from build123d import *

# Parameters (mm, degrees)
CUT_EXTRUDE1_DEPTH       = 35
SKETCH3_R                = 6.25
CUT_EXTRUDE2_DEPTH       = 35
BOSS_EXTRUDE1_REACH      = 79.604
BOSS_EXTRUDE1_END_RADIUS = 23.432556387
SKETCH4_R                = 7.25
SKETCH4_R_2              = 6.25


with BuildPart() as part:
    # Sketch1 → Revolve1 (revolve)
    with BuildSketch(Plane.XY, mode=Mode.PRIVATE) as revolve1_sk:
        with BuildLine():
            Line((25.432556387, 0), (25.432556387, 41.5))
            Line((25.432556387, 41.5), (22.932556387, 41.5))
            Line((22.932556387, 41.5), (22.932556387, 44))
            Line((22.932556387, 44), (25.432556387, 44))
            Line((25.432556387, 44), (25.432556387, 47))
            Line((25.432556387, 47), (22.932556387, 47))
            Line((22.932556387, 47), (22.932556387, 49.5))
            Line((22.932556387, 49.5), (25.432556387, 49.5))
            Line((25.432556387, 49.5), (25.432556387, 54.5))
            ThreePointArc((25.432556387, 54.5), (13.510221664, 61.275659188), (0, 63.626304471))
            Line((0, 63.626304471), (0, 61.626304471))
            ThreePointArc((0, 61.626304471), (12.394048382, 59.548269405), (23.432556387, 53.541439456))
            Line((23.432556387, 53.541439456), (23.432556387, 51.5))
            Line((23.432556387, 51.5), (20.932556387, 51.5))
            Line((20.932556387, 51.5), (20.932556387, 45.5))
            Line((20.932556387, 45.5), (20.932556387, 39.5))
            Line((20.932556387, 39.5), (23.432556387, 39.5))
            Line((23.432556387, 39.5), (23.432556387, 0))
            Line((23.432556387, 0), (25.432556387, 0))
        make_face()
    revolve(revolve1_sk.sketch.rotate(Axis((0, 0, 0), (0, 1, 0)), 90), axis=Axis((0, 0, 0), (0, 1, 0)))

    # Sketch2 → Cut-Extrude1 (cut, symmetric)
    with BuildSketch(Plane(origin=(0, 0, 0), x_dir=(0, 0, -1), z_dir=(1, 0, 0))):
        with BuildLine():
            Line((-19, 0), (19, 0))
            ThreePointArc((19, 0), (0, 10), (-19, 0))
        make_face()
    extrude(amount=CUT_EXTRUDE1_DEPTH, both=True, mode=Mode.SUBTRACT)

    # Sketch3 → Cut-Extrude2 (cut, symmetric)
    with BuildSketch(Plane.XY):
        with Locations((0, 31.626304471)):
            Circle(SKETCH3_R)
    extrude(amount=CUT_EXTRUDE2_DEPTH, both=True, mode=Mode.SUBTRACT)

    # Boss-Extrude1: up to this cylinder (the profile starts inside it)
    boss_extrude1_end = Plane(origin=(0, 31.626304, 0), z_dir=(0, -1, 0)) * Cylinder(BOSS_EXTRUDE1_END_RADIUS, 207.073112775, mode=Mode.PRIVATE)
    # Sketch4 → Boss-Extrude1 (add, up to the surface)
    with BuildSketch(Plane.XY.offset(11), mode=Mode.PRIVATE) as boss_extrude1_sk1:
        with Locations(Location((0, 31.626304471, 0), (0, 0, 180))):
            Circle(SKETCH4_R)
        with Locations((0, 31.626304471)):
            Circle(SKETCH4_R_2, mode=Mode.SUBTRACT)
    boss_extrude1_tool1 = extrude(boss_extrude1_sk1.sketch, amount=BOSS_EXTRUDE1_REACH, mode=Mode.PRIVATE) & boss_extrude1_end
    boss_extrude1 = boss_extrude1_tool1.solids().sort_by_distance((7.044939, 31.626304, 11))[0]
    add(boss_extrude1)

    # Mirror1: Boss-Extrude1 across plane
    add(boss_extrude1.mirror(Plane.XY))


solid = part.part
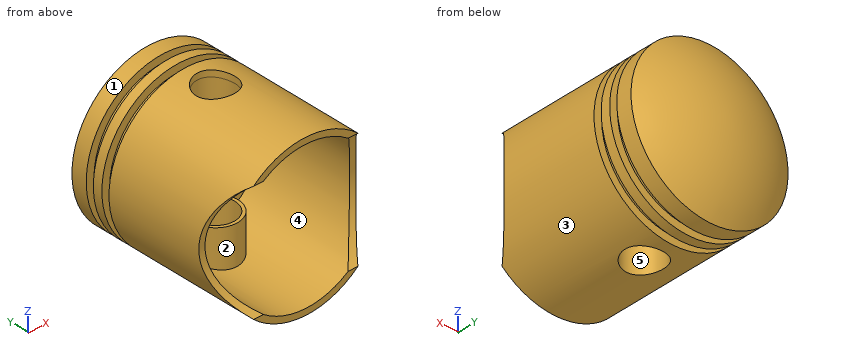
Part model, mm, in its own coordinate system. Face numbers are marked on the shaded views. A direction names the side the tool comes from. Coordinates: 2 decimals unless noted, no trailing zeros. Use a Markdown table: item, result. Add a question column.
Q1. Cut at A-A (z = 13.5). Give the number of separate pieces and of enclosed holes in the cut face, and give its area (3 significant figures).
Q2. Probe L1, parallel to X at y = 52.7, z = 0; L2, parallel to Y at x = 0, z = 24.2; L3, parallel to Y at x = 0, z = 24. List the from-to ranges inside material, lowest first.
Q3. Pin check, flat tips, straight feed: P1, Ø6, axis at x = -17, y = 10.5, coming from the +Z side; P2, Ø15.5, axis at x = 9, z = -3, coming from the -Y side; P3, Ø6, axis at x = -18.5, y = 24.5, coming from the -Z side; P4, Ø15.5, axis at x = 1, z = 1, coming from the +Y side. Stop position of each tip, or through.
Q4. Mould opens along Z. For the marked faces 3, 4 and 5 say: +Z half, -Z half, draft (parallel to the pull), parting line (faces both ways), or undercut.
Q5. Which spindle directions (+Z, -Z, +X, -X, +Y, -Y) get a long thin tool onto all of the face, cutting with end or side? Do the marked faces 1 and 2. Say none if no direction does.
Worked out:
| question | item | result |
|---|---|---|
| 1 | separate pieces | 2 |
| 1 | enclosed holes | 1 |
| 1 | area | 412 mm2 |
| 2 | L1 | x = -25.43 to -23.43, 23.43 to 25.43 |
| 2 | L2 | y = 0 to 25.38, 37.88 to 41.5, 44 to 47, 49.5 to 55.48 |
| 2 | L3 | y = 0 to 25.38, 37.88 to 41.5, 44 to 47, 49.5 to 55.63 |
| 3 | P1 | stops at z = 21.23 |
| 3 | P2 | stops at y = 57.49 |
| 3 | P3 | stops at z = -20.16 |
| 3 | P4 | stops at y = 63.63 |
| 4 | face 3 | parting line |
| 4 | face 4 | undercut |
| 4 | face 5 | draft |
| 5 | face 1 | +Y, -Y |
| 5 | face 2 | none |
